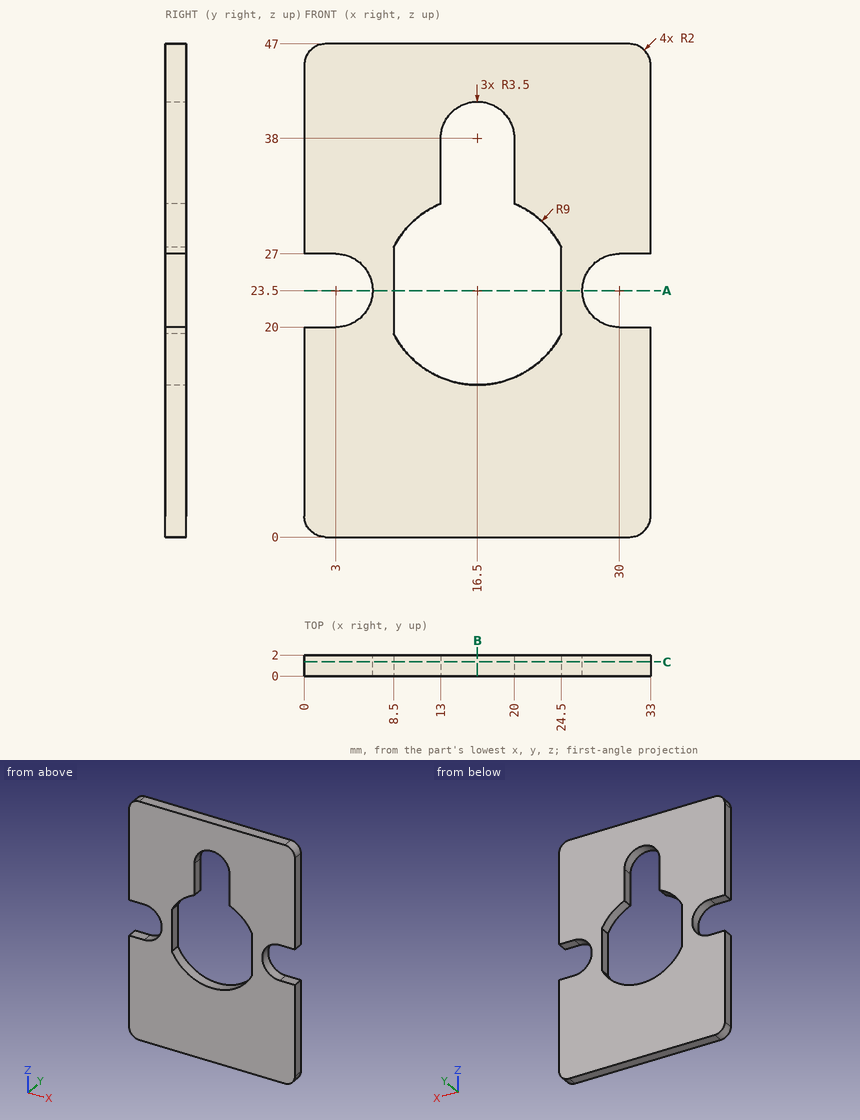
Design review of the part shown in the three views and the two pictorial views. Dimensions are in mm from the part's minimum x, y and z. Coordinates: 2 decimals unless noted, no trailing zeros. Write each loop counter-clockwise with the first axis right and the second up, starting at its lowest first coordinate (ties: lowest second). Pieces come first, ordered by that corner, then holes.
(1) Add section B-B on x = 16.5. Give the boundary of the cut face in (y, z).
(2) Add section A-A on z = 23.5. Give the boundary of the cut face in (x, y), then the cut area to 3 significant figures.
(3) Add section C-C on y = 1.35. Give the boundary of the cut face in (x, z), then the cut area to 3 significant figures.
(4) For pin 1 Ø0.6 at (y, z) = (1, 25) entering from -X; pin 2 Ø1 at (x, y) = (1, 1) entering from +Z, all flat-tipped, find the tip position at first contact; note any pin that passes through.
(5) Wall thickness on probe 1 along X at (y, z) = (0.8, 38); probe 2 along X at (y, z) = (0.5, 27.5); probe 3 along Z at (x, y) = (16.5, 0.5): over which ranges is each line inside the solid? List them lowest first.
Answer sheet:
1. outline: (0, 0) - (2, 0) - (2, 14.5) - (0, 14.5) - close; (0, 41.5) - (2, 41.5) - (2, 47) - (0, 47) - close
2. outline: (6.5, 0) - (8.5, 0) - (8.5, 2) - (6.5, 2) - close; (24.5, 0) - (26.5, 0) - (26.5, 2) - (24.5, 2) - close
2. area: 8.00 mm2
3. outline: (0, 2) arc R2 ccw to (2, 0) - (31, 0) arc R2 ccw to (33, 2) - (33, 20) - (30, 20) arc R3.5 cw to (30, 27) - (33, 27) - (33, 45) arc R2 ccw to (31, 47) - (2, 47) arc R2 ccw to (0, 45) - (0, 27) - (3, 27) arc R3.5 cw to (3, 20) - (0, 20) - close; hole (8.5, 19.38) arc R9 ccw to (24.5, 19.38) - (24.5, 27.62) arc R9 ccw to (20, 31.79) - (20, 38) arc R3.5 ccw to (13, 38) - (13, 31.79) arc R9 ccw to (8.5, 27.62) - close
3. area: 1,160 mm2
4. pin 1: stops at x = 6
4. pin 2: stops at z = 46.94
5. probe 1: x = 0 to 13, 20 to 33
5. probe 2: x = 0 to 8.5, 24.5 to 33
5. probe 3: z = 0 to 14.5, 41.5 to 47
